The drawing under review shows one solid part. Ordinate dimensions are in mm from its lowest x, y, z. A direction names the side the tool comes from. Give positions to 0.01 mm unless a question says otherwise; leave off trailing zeros. Order: outer loops, then holes, each group sorted by start corner. A loop starts at its lowest first (then second) coordinate and runs counter-clockwise, first axis right, second up. Notation, with made-up numbers: (-8, 23) -> (48, 23) arc R19 ccw to (48, 34) -> close; hole circle Ø2 at (-29, 89). An arc over 180 degrees is marked (long way). One line per item, written item: value. Start each with the question number.
1) For pin 1 (3 mm diameter, centred on x = 9.5, y = 5, fed in from -Z), flat-tipped, find the tip position at first contact; note if it passes through.
2) The part is to be moulded in two halves that separate along X. For the marked faces 3, 4 and 5, say which applies: released by +X, released by -X, zero draft, split by the parting line, or undercut.
3) Consider section A-A (x = 2). State the section outline as (y, z) points (1 decimal).
4) Tool access review of the marked faces 1 and 2: name each direction out of +Z, -Z, +X, -X, +Y, -Y from which nothing blocks a thin tool from reaching the whole face with its end or side.
5) Wall thickness on line 1 along X through (y, z) = (5.5, 5) (1 decimal); line 2 along X through (y, z) = (1.25, 5.5) (1 decimal); line 3 along Y through (x, z) = (13, 3.25): over which ranges is each line inside the solid? List them lowest first. Write a range as from..to.
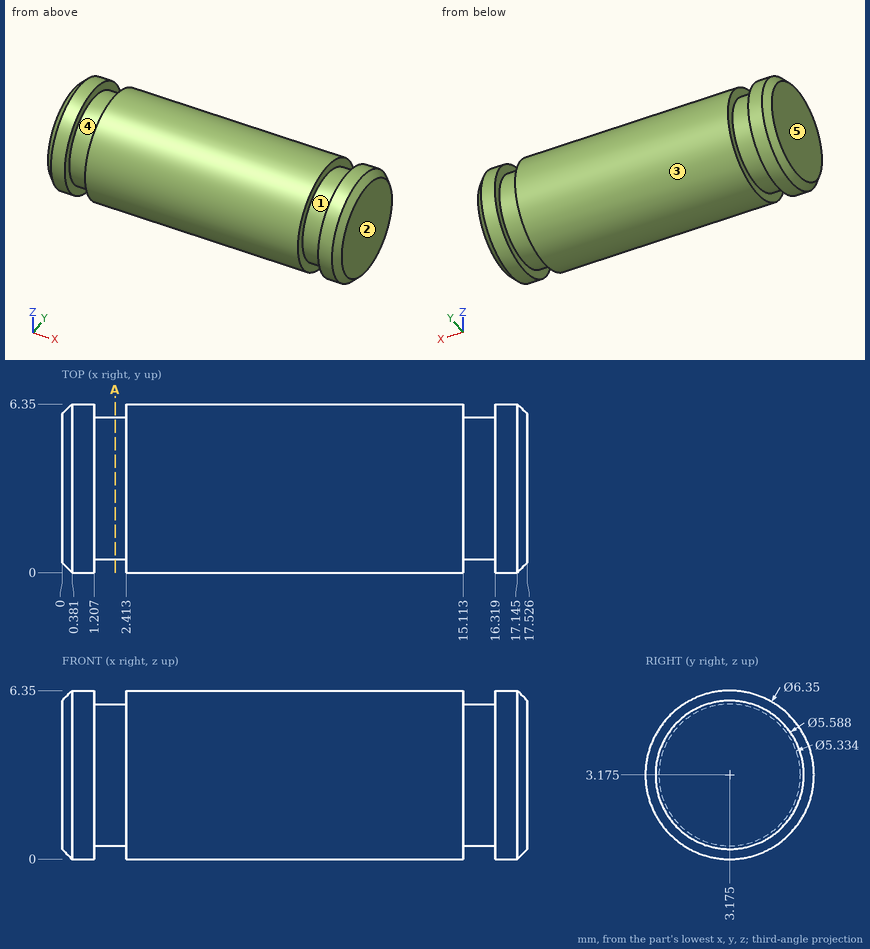
Checked values:
1. pin 1: stops at z = 0.02
2. face 3: zero draft
2. face 4: undercut
2. face 5: released by -X
3. outline: circle Ø5.3 at (3.2, 3.2)
4. face 1: none
4. face 2: +Z, -Z, +X, +Y, -Y
5. line 1: x = 0.2..1.2, 2.4..15.1, 16.3..17.4
5. line 2: x = 0.2..1.2, 2.4..15.1, 16.3..17.3
5. line 3: y = 0..6.35
